Input: part model. Units: mm. Frame: model coordinates. Give positions to 0.01 mm unless a question says otherwise; leave off trailing zeros. Write each loop counter-clockwise with the first axis right and the second up, starting at its lowest first coordinate (ties: lowest second). Pieces come first, ordered by that corner, then holes. Notation, with made-up numbers: (-1.75, 86) -> (9.25, 86) arc R20 cw to (9.25, 103) -> close; hole circle Ø1 at (89, 84.25). An arc over 180 degrees is marked (long way). Return JSON: item names as keys, results as strings. Group by question number.
Item 1: Section B-B, the plane z = 0. Return loops of the section in (x, y) (3 decimals), then the cut area to 3 significant figures.
Item 2: Section C-C, the plane x = 0. Return loops of the section in (y, z) (3 decimals).
Item 3: Mould query, pull axis Z, two halves, no side actions, for faces 1 (the face through (-9.525, -67, -4)), 2 (the face through (0.133, -74.107, 1.409)), 3 (the face through (-15.12, -11.59, 0.76)). Classes: released by +Z, released by -Z, zero draft, split by the parting line, or undercut.
Item 4: Pin query (flat end, axial travel): P1, Ø1.5, axis at x = -12, z = -0.5, coming from the +Y side; P2, Ø2, axis at x = -1.5, y = -49, coming from the -Z side; P3, Ø11.5, axis at x = 5.5, y = -5, coming from the +Z side; P4, Ø3.5, axis at y = -70.06, z = 0, coming from the +X side. Return the tip coordinate at first contact, or that it passes through.
Item 5: Section A-A, the plane y = -32. Return loops of the section in (x, z) (3 decimals).
Item 6: Line query: line 1 (Z direction, x = 4.5, y = -60.5); line 2 (Y direction, x = -1, z = 6.5); line 3 (Y direction, x = 5, z = -35.5). Output: solid intervals per line, ascending. Write a range as [from, to].
Item 7: Section D-D, the plane z = -40. Return loops of the section in (x, y) (3 decimals).
from build123d import *

# Parameters (mm, degrees)
F0_R     = 19.05
F1_DEPTH = 53.975
F2_R     = 2.831223
F3_DEPTH = 9.525


with BuildPart() as f1:
    # F0 (on Top) → F1 (new body, symmetric)
    with BuildSketch(Plane.XY):
        Circle(F0_R)
    extrude(amount=F1_DEPTH, both=True)

    # F2 (on Right) → F3 (join, symmetric)
    with BuildSketch(Plane.YZ):
        with BuildLine():
            Line((0, -54.249428), (0, 54.076027))
            ThreePointArc((0, 54.076027), (-74.126923, -0.086701), (0, -54.249428))
        make_face()
        with Locations((-70.061542, 0)):
            Circle(F2_R, mode=Mode.SUBTRACT)
        with BuildLine():
            ThreePointArc((-14.80739, -54.97568), (-65.170353, -0.086549), (-14.807088, 54.802305))
            Line((-14.807088, 54.802305), (-14.807088, 54.076027))
            Line((-14.807088, 54.076027), (-14.807088, -54.249428))
            Line((-14.807088, -54.249428), (-14.80739, -54.97568))
        make_face(mode=Mode.SUBTRACT)
    extrude(amount=F3_DEPTH, both=True)


solid = f1.part
Answer below:
{
 "1": {"outline": "circle Ø38.1 at (0, 0); (-9.525, -74.127) -> (9.525, -74.127) -> (9.525, -72.893) -> (-9.525, -72.893) -> close; (-9.525, -67.23) -> (9.525, -67.23) -> (9.525, -65.17) -> (-9.525, -65.17) -> close", "area": "1,200 mm2"},
 "2": {"outline": "(0, -54.249) -> (0, -53.975) -> (19.05, -53.975) -> (19.05, 53.975) -> (0, 53.975) -> (0, 54.076) arc R56.851 ccw (long way) to start; hole circle Ø5.662 at (-70.062, 0); hole (-19.05, -53.975) -> (-19.05, 53.975) -> (-14.807, 53.975) -> (-14.807, 54.802) arc R55.092 ccw to (-14.807, -54.976) -> (-14.807, -54.249) -> (-14.807, -53.975) -> close"},
 "3": {"face 1": "zero draft", "face 2": "split by the parting line", "face 3": "undercut"},
 "4": {"P1": "stops at y = 15.37", "P2": "stops at z = -47.92", "P3": "stops at z = 56.39", "P4": "passes through"},
 "5": {"outline": "(-9.525, -54.998) -> (9.525, -54.998) -> (9.525, -50.63) -> (-9.525, -50.63) -> close; (-9.525, 50.456) -> (9.525, 50.456) -> (9.525, 54.825) -> (-9.525, 54.825) -> close"},
 "6": {"line 1": "z = [-37.02, -22.29], [22.11, 36.84]", "line 2": "y = [-73.74, -64.78], [-19.02, 19.02]", "line 3": "y = [-61.75, -52.28], [-18.38, 18.38]"},
 "7": {"outline": "circle Ø38.1 at (0, 0); (-9.525, -57.76) -> (9.525, -57.76) -> (9.525, -48.053) -> (-9.525, -48.053) -> close"}
}
